Source: CAD feature listing. Evaluate the final solid. Frame: model axes, mm. Face numbers are marked on the shaded views. A direction names the side the tool comes from. Round coordinates to 2 decimals unless told otherwise and drop trailing zeros. Loops run counter-clockwise (first coordinate to the right, second up) from the corner with the lowest first, then second, coordinate; pieces in that order, holes last. Notation, with made-up numbers: M -28.75,-4.75 L -24.75,-4.75 A25 cw -24.75,15.25 Z; hole C 6,18.5 d3. An arc over 180 degrees is marked long. Write each question's results on one line, items separated by ' | '. Start each with the question number.
1. Contact query for flat-ended pins moving along their axis: pin 1 Ø5 at (y, z) = (6.5, 12) entering from +X; pin 2 Ø10 at (x, y) = (-1, 4.5) entering from -Z; pin 3 Ø1 at (y, z) = (-0.5, 58) entering from -X; pin 4 Ø10 at (x, z) = (-2, 46) entering from +Y. Output: stop coordinate, or through.
2. Section A-A on y = 0. Output: boundary loops of the cut face in (x, z).
3. Section C-C on z = 55. Output: boundary loops of the cut face in (x, y).
4. Ray query, line 1 (Z direction, x = -7.25, y = -4.25); line 2 (Z direction, x = 2, y = -1.5); line 3 (X direction, y = 4.25, z = 21.5). Return the intervals inside material, ascending.
5. Set-up query: the marked faces 1 and 2. Return all of +Z, -Z, +X, -X, +Y, -Y with unobstructed straight access to the full face (end or side cutting, diameter ignored); none if empty.
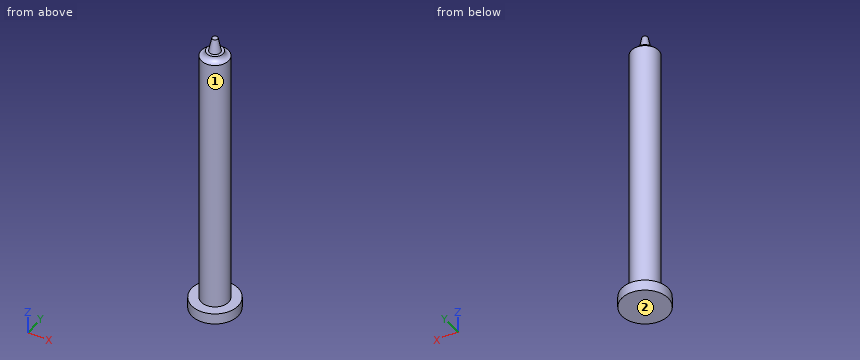
from build123d import *

# Parameters (mm, degrees)
F0_R     = 8.5
F1_DEPTH = 4
F2_R     = 5
F3_DEPTH = 100


with BuildPart() as f1:
    # F0 (on Top) → F1 (new body)
    with BuildSketch(Plane.XY):
        Circle(F0_R)
    extrude(amount=F1_DEPTH)

    # F2 (on Top) → F3 (join)
    with BuildSketch(Plane.XY):
        Circle(F2_R)
    extrude(amount=F3_DEPTH)

    # F4 (on Right) → F5 (revolve)
    with BuildSketch(Plane.YZ):
        with BuildLine():
            Line((3, 102), (0, 102))
            Line((0, 102), (0, 100))
            Line((0, 100), (5, 100))
            ThreePointArc((5, 100), (3.585786, 100.585786), (3, 102))
        make_face()
    revolve(axis=Axis((0, 0, 101), (0, 0, -1)))

    # F6 (on Right) → F7 (revolve)
    with BuildSketch(Plane.YZ):
        Polygon((0, 107), (0, 102), (2, 102), (1, 107), align=None)
    revolve(axis=Axis((0, 0, 104.5), (0, 0, 1)))


solid = f1.part
Taken from the geometry:
1) pin 1: x = 3 | pin 2: z = 0 | pin 3: x = -5 | pin 4: y = 5
2) outline: M -8.5,0 L 8.5,0 L 8.5,4 L 5,4 L 5,100 A2 cw 3,102 L 2,102 L 1,107 L -1,107 L -2,102 L -3,102 A2 cw -5,100 L -5,4 L -8.5,4 Z
3) outline: C 0,0 d10
4) line 1: 0 to 4 | line 2: 0 to 102 | line 3: -2.63 to 2.63
5) face 1: +Z | face 2: -Z, +X, -X, +Y, -Y
